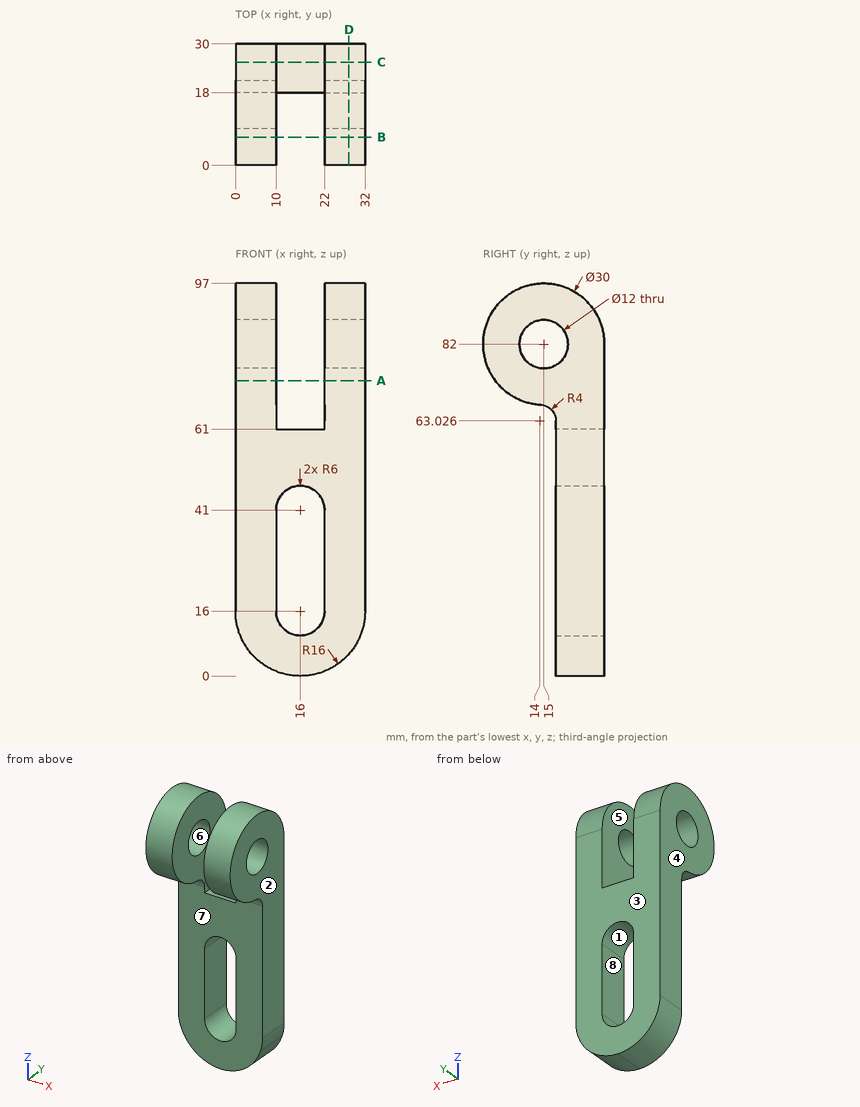
Design review of the part shown in the three views and the two pictorial views. Dimensions are in mm from the part's minimum x, y and z. A direction names the side the tool comes from. Round coordinates to 2 decimals unless told otherwise and drop trailing zeros. Write each loop counter-clockwise with the first axis right and the second up, starting at its lowest first coordinate (ties: lowest second). Pieces come first, ordered by that corner, then holes. Notation, with made-up numbers: (-10, 84) -> (0, 84) arc R18 cw to (0, 107) -> close; hole circle Ø5 at (9.5, 88.25). An arc over 180 degrees is marked (long way). One line per question, with ' | ' between items. Start each with the question number.
1) Mouldability with a two-part tool opening along X and no side actions: class the marked faces 1, 2, 3 and 4 as +X half, -X half, draft (parallel to the pull), parting line (faces both ways), or undercut.
2) Add section D-D (x = 28). Write out the cut boundary in (y, z).
3) For pin 1 Ø5 at (x, y) = (4, 4) entering from +Z; pin 2 Ø2 at (x, z) = (28.5, 30.5) entering from -Y; pin 3 Ø4 at (x, y) = (6.5, 11.5) entering from -Z (1 decimal), all flat-tipped, find the tip position at first contact; note any pin that passes through.
4) Machinability: for the marked faces 5, 6, 7 and 8, which of the approach directions +Z, -Z, +X, -X, +Y, -Y give a long, thin tool a straight path to every point of the face, cutting with its end or side? Answer none if there is none.
5) Add section C-C (y = 25.5). Write out the cut boundary in (x, z).
6) Wall thickness on line 1 along Y through (x, z) = (25, 82); line 2 along X through (y, z) = (28.25, 64.5); line 3 along Y through (x, z) = (25, 31): over which ranges is each line inside the solid? List them lowest first.
7) Add section B-B (y = 7). Write out the cut boundary in (x, z).
8) Add section A-A (z = 73). Write out the cut boundary in (x, y), and give its area (3 significant figures).
Reported:
1) face 1: undercut | face 2: +X half | face 3: draft | face 4: -X half
2) outline: (14.21, 67.02) arc R4 cw to (18, 63.03) -> (18, 5.42) -> (30, 5.42) -> (30, 82) arc R15 ccw (long way) to start; hole circle Ø12 at (15, 82)
3) pin 1: stops at z = 94.36 | pin 2: stops at y = 18 | pin 3: stops at z = 67.1
4) face 5: +Z, +Y, -Y | face 6: +X, -X | face 7: -Z, +X, -X, -Y | face 8: +Y, -Y
5) outline: (0, 16) arc R16 ccw to (32, 16) -> (32, 92.71) -> (22, 92.71) -> (22, 61) -> (10, 61) -> (10, 92.71) -> (0, 92.71) -> close; hole (10, 16) arc R6 ccw to (22, 16) -> (22, 41) arc R6 ccw to (10, 41) -> close
6) line 1: y = 0 to 9, 21 to 30 | line 2: x = 0 to 10, 22 to 32 | line 3: y = 18 to 30
7) outline: (0, 69.31) -> (10, 69.31) -> (10, 94.69) -> (0, 94.69) -> close; (22, 69.31) -> (32, 69.31) -> (32, 94.69) -> (22, 94.69) -> close
8) outline: (0, 3) -> (10, 3) -> (10, 30) -> (0, 30) -> close; (22, 3) -> (32, 3) -> (32, 30) -> (22, 30) -> close | area: 540 mm²
